```python
from build123d import *

# Parameters (mm, degrees)
SKETCH1_W                   = 25.4
SKETCH1_H                   = 50.8
BOSS_EXTRUDE1_DEPTH         = 154.94
SHELL1_T                    = -1.5875
F_21_0_159_DIAMETER_HOLE1_D = 4.0386
LPATTERN1_COUNT             = 11
LPATTERN1_PITCH             = 12.7
LPATTERN1_COUNT_DIR2        = 2
LPATTERN1_PITCH_DIR2        = 25.4
F_1_2_0_5_DIAMETER_HOLE1_D  = 12.7
LPATTERN2_COUNT             = 5
LPATTERN2_PITCH             = 25.4
F_21_0_159_DIAMETER_HOLE2_D = 4.0386
LPATTERN3_COUNT             = 11
LPATTERN3_PITCH             = 12.7


with BuildPart() as part:
    # Sketch1 → Boss-Extrude1 (new body)
    with BuildSketch(Plane.XY):
        with Locations((12.7, 25.4)):
            Rectangle(SKETCH1_W, SKETCH1_H)
    extrude(amount=BOSS_EXTRUDE1_DEPTH)

    # Shell1
    shell1_openings = [part.faces().sort_by_distance(p)[0] for p in [
        (12.7, 25.4, 154.94),
        (12.7, 25.4, 0),
    ]]
    offset(amount=SHELL1_T, openings=shell1_openings, kind=Kind.INTERSECTION)

    # #21 (0.159) Diameter Hole1 (through all)
    with Locations(Plane(origin=(25.4, 0, 0), x_dir=(0, 0, -1), z_dir=(1, 0, 0))):
        with Locations((-12.7, 38.1)):
            f_21_0_159_diameter_hole1 = Hole(F_21_0_159_DIAMETER_HOLE1_D / 2)

    # LPattern1: 21 _0.159_ Diameter Hole1 11 × 2
    with Locations(*[(0, -j * LPATTERN1_PITCH_DIR2, i * LPATTERN1_PITCH) for i in range(LPATTERN1_COUNT) for j in range(LPATTERN1_COUNT_DIR2) if (i, j) != (0, 0)]):
        add(f_21_0_159_diameter_hole1, mode=Mode.SUBTRACT)

    # 1/2 (0.5) Diameter Hole1 (through all)
    with Locations(Plane(origin=(25.4, 0, 0), x_dir=(0, 0, -1), z_dir=(1, 0, 0))):
        with Locations((-19.05, 25.4)):
            f_1_2_0_5_diameter_hole1 = Hole(F_1_2_0_5_DIAMETER_HOLE1_D / 2)

    # LPattern2: 1/2 (0.5) Diameter Hole1 ×5
    with Locations(*[(0, 0, i * LPATTERN2_PITCH) for i in range(1, LPATTERN2_COUNT)]):
        add(f_1_2_0_5_diameter_hole1, mode=Mode.SUBTRACT)

    # #21 (0.159) Diameter Hole2 (through all)
    with Locations(Plane(origin=(0, 50.8, 0), x_dir=(1, 0, 0), z_dir=(0, 1, 0))):
        with Locations((12.7, -12.7)):
            f_21_0_159_diameter_hole2 = Hole(F_21_0_159_DIAMETER_HOLE2_D / 2)

    # LPattern3: #21 (0.159) Diameter Hole2 ×11
    with Locations(*[(0, 0, i * LPATTERN3_PITCH) for i in range(1, LPATTERN3_COUNT)]):
        add(f_21_0_159_diameter_hole2, mode=Mode.SUBTRACT)


solid = part.part
```
Can you work these out from the model? Positions are in its coordinate system, mm. A direction names the side the tool comes from. Coordinates: 2 decimals unless noted, no trailing zeros. Loops run counter-clockwise (first coordinate to the right, second up) from the corner with the lowest first, then second, coordinate; pieces in that order, holes last. Notation, with made-up numbers: (-9, 46.5) - (15, 46.5) arc R13 cw to (15, 51.5) - close; hole circle Ø9 at (17, 2). An arc over 180 degrees is marked (long way). Use a Markdown table: item, result.
Item 1: For faces 3 (the face through (24.595, 22.968, 50.316)), 4 (the face through (23.812, 25.1, 76.4)), which set-ups out of +Z, -Z, +X, -X, +Y, -Y let a thin tool reach every point of the face, with its end or its side?
Numbers:
| item | result |
|---|---|
| face 3 | +X, -X |
| face 4 | +Z, -Z |
Item 2: I want a section at D-D on z = 69.85. Please give me the cut outline in (x, y).
Numbers:
| item | result |
|---|---|
| outline | (0, 0) - (25.4, 0) - (25.4, 19.05) - (23.81, 19.05) - (23.81, 1.59) - (1.59, 1.59) - (1.59, 19.05) - (0, 19.05) - close; (0, 31.75) - (1.59, 31.75) - (1.59, 49.21) - (23.81, 49.21) - (23.81, 31.75) - (25.4, 31.75) - (25.4, 50.8) - (0, 50.8) - close |
Item 3: We'd pull the mould along Z, two halves only. Please class faces 1 (the face through (15, 0, 76)), 2 (the face through (12.963, 0.783, 99.598)): released by +Z, released by -Z, zero draft, split by the parting line, or undercut.
Numbers:
| item | result |
|---|---|
| face 1 | zero draft |
| face 2 | undercut |
Item 4: I want a section at A-A on z = 139.7. Give the number of separate pieces and of enclosed holes in the cut face, and give its area (3 significant figures).
Numbers:
| item | result |
|---|---|
| separate pieces | 6 |
| enclosed holes | 0 |
| area | 193 mm2 |
Item 5: I want a section at B-B on y = 42. Please give me the cut outline in (x, z), and give its area (3 significant figures).
Numbers:
| item | result |
|---|---|
| outline | (0, 0) - (1.59, 0) - (1.59, 154.94) - (0, 154.94) - close; (23.81, 0) - (25.4, 0) - (25.4, 154.94) - (23.81, 154.94) - close |
| area | 492 mm2 |
Item 6: I want a section at C-C on x = 16.5. Please give me the cut outline in (y, z), and give its area (3 significant figures).
Numbers:
| item | result |
|---|---|
| outline | (0, 0) - (1.59, 0) - (1.59, 154.94) - (0, 154.94) - close; (49.21, 0) - (50.8, 0) - (50.8, 154.94) - (49.21, 154.94) - close |
| area | 492 mm2 |
Item 7: Will this pin go through, and if not, where does the flat tip stop? pin 1 (1.5 mm diameter, centred on x = 14.5, z = 61, fed in from -Y).
Numbers:
| item | result |
|---|---|
| pin 1 | stops at y = 0 |
Item 8: If I drill on probe 1 along Y at (x, z) = (18.5, 22); probe 2 along Z at (x, y) = (24.25, 24.5); probe 3 along X at (y, z) = (48.5, 130.5), over which ranges is the centre line in solid material (lowest first)? Write a range as from..to.
Numbers:
| item | result |
|---|---|
| probe 1 | y = 0..1.59, 49.21..50.8 |
| probe 2 | z = 0..12.76, 25.34..38.16, 50.74..63.56, 76.14..88.96, 101.54..114.36, 126.94..154.94 |
| probe 3 | x = 0..1.59, 23.81..25.4 |
